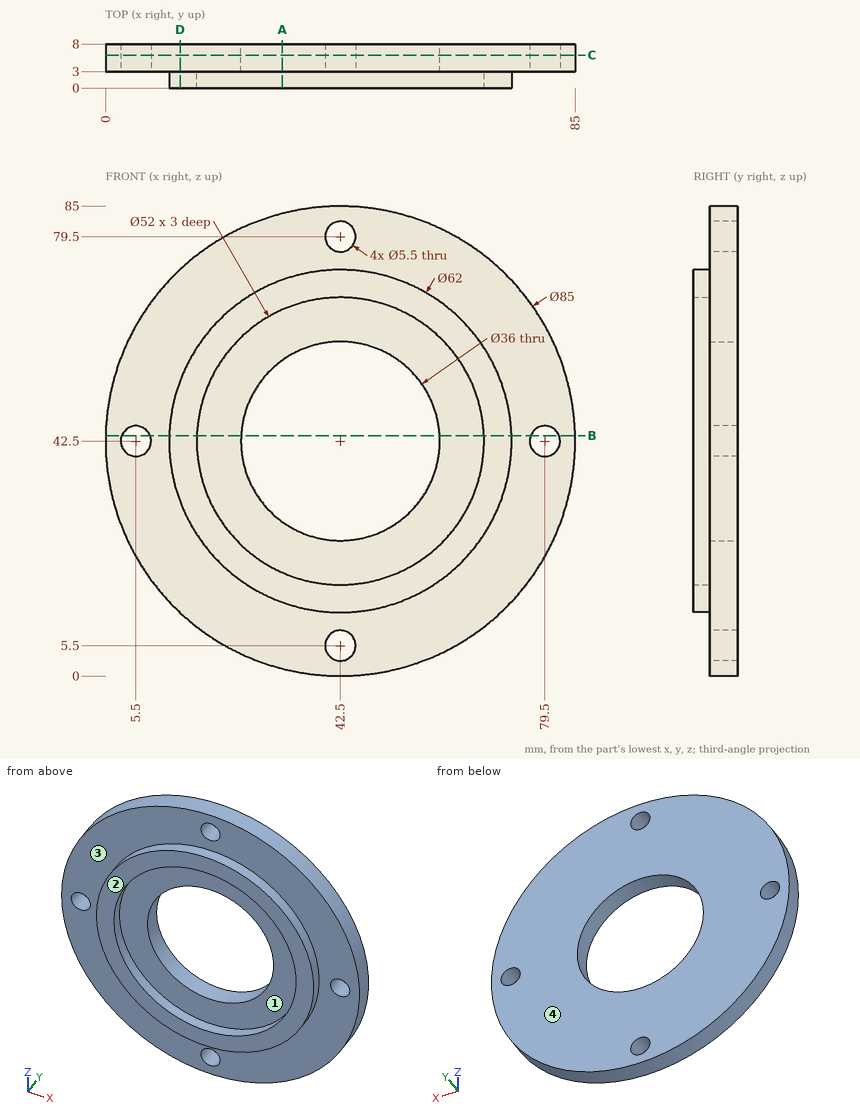
Input: dimensioned drawing with shaded views. Units: mm. Origin: part minimum x, y, z. A direction names the side the tool comes from. Give positions to 0.01 mm unless a question says otherwise; leave off trailing zeros. Order: outer loops, then holes, each group sorted by start corner. A loop starts at its lowest first (then second) coordinate and runs counter-clockwise, first axis right, second up. Notation, with made-up numbers: (66.25, 85.5) -> (122.25, 85.5) arc R27 ccw to (122.25, 117.5) -> close; hole circle Ø7 at (-6, -12.5). An arc over 180 degrees is marked (long way). Use one line per item in the form item = value.
1) First-contact query: pin 1 Ø5 at (x, z) = (42.5, 79.5) entering from -Y; pin 2 Ø2 at (x, y) = (32.5, 1.5) entering from -Z; pin 3 Ø2 at (x, y) = (36, 6.5) entering from -Z; pin 4 Ø1.5 at (y, z) = (1, 39.5) entering from -X. Flat tips, straight axial feed; report the tip coordinate or a pass-through.
Response values:
pin_1 = through
pin_2 = 12.84
pin_3 = 0.36
pin_4 = 11.58
2) Mould query, pull axis X, two halves, no side actions, for the marked faces 1 and 2. Classes: pulls with the +X half, pulls with the -X half, needs draft (parallel to the pull), parting line crosses it, or undercut.
Response values:
face_1 = undercut
face_2 = needs draft
3) Section D-D, the plane x = 13.5. Return loops of the section in (y, z).
Response values:
outline = (0, 31.55) -> (3, 31.55) -> (3, 11.43) -> (8, 11.43) -> (8, 73.57) -> (3, 73.57) -> (3, 53.45) -> (0, 53.45) -> close
4) Line query: probe 1 along X at (y, z) = (5.15, 42.5); probe 2 along X at (y, z) = (2.2, 42.5). Output: solid intervals per line, ascending.
Response values:
probe_1 = 0 to 2.75, 8.25 to 24.5, 60.5 to 76.75, 82.25 to 85
probe_2 = 11.5 to 16.5, 68.5 to 73.5
5) Section A-A, the plane x = 32. Return loops of the section in (y, z), and give its area (3 significant figures).
Response values:
outline = (0, 13.33) -> (3, 13.33) -> (3, 1.32) -> (8, 1.32) -> (8, 27.88) -> (3, 27.88) -> (3, 18.71) -> (0, 18.71) -> close; (0, 66.29) -> (3, 66.29) -> (3, 57.12) -> (8, 57.12) -> (8, 83.68) -> (3, 83.68) -> (3, 71.67) -> (0, 71.67) -> close
area = 298 mm^2
6) Section C-C, the plane y = 6. Return loops of the section in (x, z), and give its area (3 significant figures).
Response values:
outline = circle Ø85 at (42.5, 42.5); hole circle Ø5.5 at (5.5, 42.5); hole circle Ø36 at (42.5, 42.5); hole circle Ø5.5 at (42.5, 5.5); hole circle Ø5.5 at (42.5, 79.5); hole circle Ø5.5 at (79.5, 42.5)
area = 4,560 mm^2
7) Section B-B, the plane z = 43.5. Return loops of the section in (x, y).
Response values:
outline = (0.01, 3) -> (2.94, 3) -> (2.94, 8) -> (0.01, 8) -> close; (8.06, 3) -> (11.52, 3) -> (11.52, 0) -> (16.52, 0) -> (16.52, 3) -> (24.53, 3) -> (24.53, 8) -> (8.06, 8) -> close; (60.47, 3) -> (68.48, 3) -> (68.48, 0) -> (73.48, 0) -> (73.48, 3) -> (76.94, 3) -> (76.94, 8) -> (60.47, 8) -> close; (82.06, 3) -> (84.99, 3) -> (84.99, 8) -> (82.06, 8) -> close
8) Reachability of the marked faces 3 and 4 from +Z, -Z, +X, -X, +Y, -Y: full face, straight path, thin tool, end or side. Return the list, or none.
Response values:
face_3 = -Y
face_4 = +Z, -Z, +X, -X, +Y
